Job drawing, mm, ordinate dimensions from the low corner. One solid piece. A direction names the side the tool comes from. Give positions to 0.01 mm unless a question says otherwise; leave off trailing zeros. Order: outer loops, then holes, each group sorted by start corner. A loop starts at its lowest first (then second) coordinate and runs counter-clockwise, first axis right, second up. Notation, with made-up numbers: (18.5, 62) -> (50.5, 62) arc R7 ccw to (50.5, 75) -> close; hole circle Ø4 at (-36.75, 20). An arc over 180 degrees is marked (long way). Use CSV: the item, a comma, the result in double quotes. Start each with the question number.
1. Drop flat-ended pins along their axis: pin 1 (2.5 mm diameter, centred on x = 25, z = 21.24, fed in from -Y); pin 2 (4 mm diameter, centred on x = 25, z = 5.16, fed in from -Y); pin 3 (5 mm diameter, centred on y = 21.5, z = 7, fed in from +X); pin 4 (4 mm diameter, centred on x = 6, z = 10, fed in from +Y). Give the stop position or say it passes through.
2. Cut at C-C on x = 14. List the corners of the cut face in (y, z), then the cut area to 3 significant figures.
3. Wall check: line 1 (Z direction, x = 11, y = 2); line 2 (X direction, y = 15, z = 5.5); line 3 (X direction, y = 1.5, z = 13.2). Give the ranges that are in metal, low to high. Write a range as from..to.
4. Cut at B-B on x = 25. List the corners of the cut face in (y, z), then the cut area to 3 significant figures.
5. Cut at A-A on y = 19.25. List the corners of the cut face in (x, z), then the cut area to 3 significant figures.
6. Pull direction Y, two halves, no side cores. Call the marked faces 1, 2 and 3: released by +Y, released by -Y, zero draft, split by the parting line, or undercut.
7. Cut at D-D on y = 10. List the corners of the cut face in (x, z), then the cut area to 3 significant figures.
8. 3-axis set-ups, long thin cutter, end or side, ignore diameter. For the marked faces 4 and 5: which of +Z, -Z, +X, -X, +Y, -Y reach the whole face in a straight line?
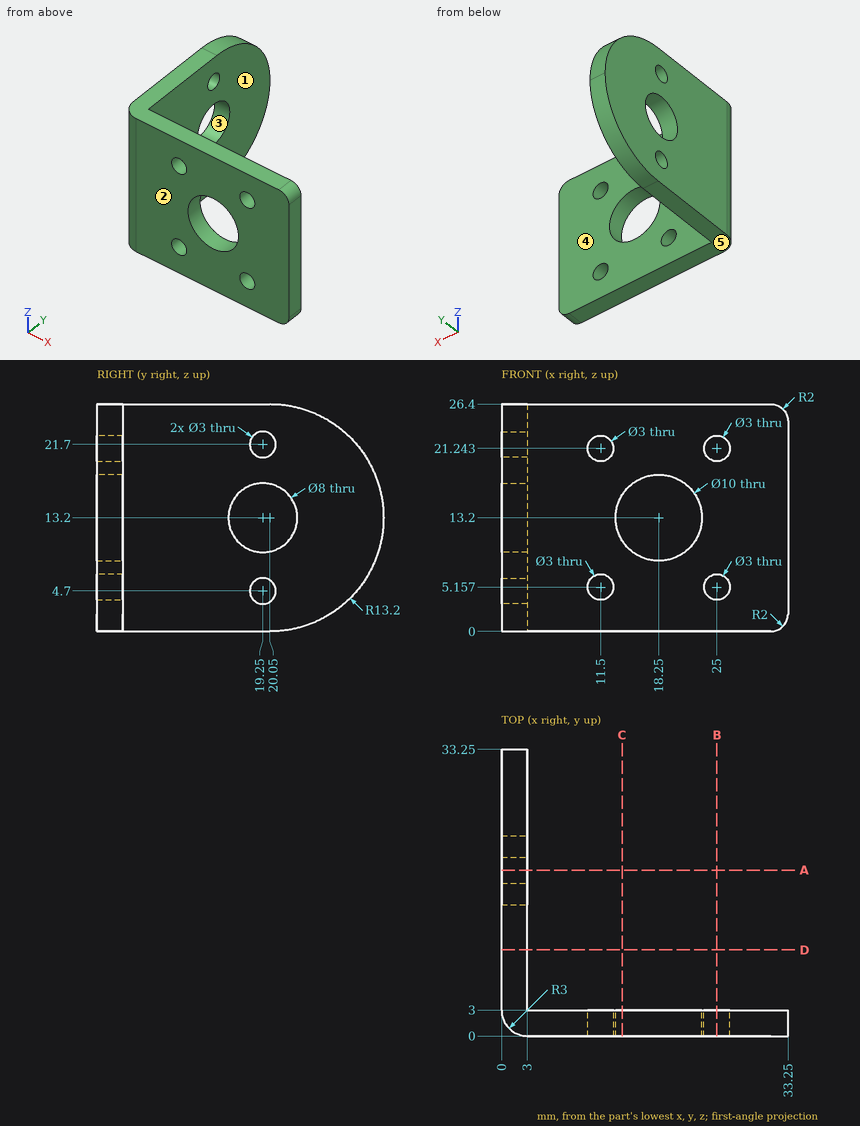
Verdict:
1,pin 1,"through"
1,pin 2,"y = 0"
1,pin 3,"x = 3"
1,pin 4,"y = 3"
2,outline,"(0, 0) -> (3, 0) -> (3, 10.57) -> (0, 10.57) -> close; (0, 15.83) -> (3, 15.83) -> (3, 26.4) -> (0, 26.4) -> close"
2,area,"63.4 mm^2"
3,line 1,"0..3.74, 6.57..19.83, 22.66..26.4"
3,line 2,"0..3"
3,line 3,"0.4..13.25, 23.25..33.25"
4,outline,"(0, 0) -> (3, 0) -> (3, 3.66) -> (0, 3.66) -> close; (0, 6.66) -> (3, 6.66) -> (3, 19.74) -> (0, 19.74) -> close; (0, 22.74) -> (3, 22.74) -> (3, 26.4) -> (0, 26.4) -> close"
4,area,"61.2 mm^2"
5,outline,"(0, 0) -> (3, 0) -> (3, 3.2) -> (0, 3.2) -> close; (0, 6.2) -> (3, 6.2) -> (3, 9.2) -> (0, 9.2) -> close; (0, 17.2) -> (3, 17.2) -> (3, 20.2) -> (0, 20.2) -> close; (0, 23.2) -> (3, 23.2) -> (3, 26.4) -> (0, 26.4) -> close"
5,area,"37.2 mm^2"
6,face 1,"zero draft"
6,face 2,"released by -Y"
6,face 3,"undercut"
7,outline,"(0, 0) -> (3, 0) -> (3, 26.4) -> (0, 26.4) -> close"
7,area,"79.2 mm^2"
8,face 4,"+Z, -Z, +X, +Y"
8,face 5,"-Z, +X, -X, +Y, -Y"
